Geometry check sheet. Reference: the model listing, model coordinates, mm. A direction names the side the tool comes from. Give positions to 0.01 mm unless a question says otherwise; leave off trailing zeros. Loops run counter-clockwise (first coordinate to the right, second up) from the corner with the lowest first, then second, coordinate; pieces in that order, holes last. Notation, with made-up numbers: (37.25, -17) -> (87.25, -17) arc R20 cw to (87.25, 15) -> close; hole circle Ø3 at (-28, 65). An arc over 180 degrees is marked (long way). One line per question, with ' | ' between items.
from build123d import *

# Parameters (mm, degrees)
ESQUISSE1_R                      = 2
ESQUISSE1_R_2                    = 1.8
ESQUISSE1_W                      = 7
ESQUISSE1_H                      = 9.3
ESQUISSE1_W_2                    = 9.3
ESQUISSE1_H_2                    = 7
BOSS_EXTRU_1_DEPTH               = 3
R_P_TITION_START                 = -3
R_P_TITION_CIRCULAIRE1_OUTLINE_R = 2
R_P_TITION_CIRCULAIRE1_DEPTH     = 6
CHANFREIN1_SIZE                  = 3
IDLER_REACH                      = 155.922
ESQUISSE2_R                      = 2.5
ESQUISSE2_W                      = 8
ESQUISSE2_H                      = 16
SCREEN_REACH                     = 155.922
ESQUISSE3_R                      = 2


# Read off the part's stored shape, not the designer's step: Répétition circulaire1
with BuildPart() as part:
    # Esquisse1 → Boss.-Extru.1 (new, symmetric)
    with BuildSketch(Plane.XY):
        with BuildLine():
            Line((-150, -26), (0, -26))
            Line((0, -26), (0, 26))
            Line((0, 26), (-4, 26))
            Line((-4, 26), (-4, 34))
            Line((-4, 34), (-81, 34))
            Line((-81, 34), (-81, 30))
            ThreePointArc((-81, 30), (-85, 26), (-89, 30))
            Line((-89, 30), (-89, 34))
            Line((-89, 34), (-98, 34))
            Line((-98, 34), (-98, 26))
            Line((-98, 26), (-118, 26))
            Line((-118, 26), (-118, 34))
            Line((-118, 34), (-150, 34))
            Line((-150, 34), (-150, -26))
        make_face()
        with Locations((-93, 28)):
            Circle(ESQUISSE1_R, mode=Mode.SUBTRACT)
        with Locations((-144, 4)):
            Circle(ESQUISSE1_R_2, mode=Mode.SUBTRACT)
        with Locations((-50, -20)):
            Circle(ESQUISSE1_R_2, mode=Mode.SUBTRACT)
        with Locations((-144, 15.65)):
            Rectangle(ESQUISSE1_W, ESQUISSE1_H, mode=Mode.SUBTRACT)
        with Locations((-144, -7.65)):
            Rectangle(ESQUISSE1_W, ESQUISSE1_H, mode=Mode.SUBTRACT)
        with Locations((-38.35, -20)):
            Rectangle(ESQUISSE1_W_2, ESQUISSE1_H_2, mode=Mode.SUBTRACT)
        with Locations((-61.65, -20)):
            Rectangle(ESQUISSE1_W_2, ESQUISSE1_H_2, mode=Mode.SUBTRACT)
    extrude(amount=BOSS_EXTRU_1_DEPTH, both=True)

    # Répétition circulaire1 outline → Répétition circulaire1 (cut)
    with BuildSketch(Plane.XY.offset(R_P_TITION_START)):
        with Locations((-77.07179677, 27.732050808)):
            Circle(R_P_TITION_CIRCULAIRE1_OUTLINE_R)
        with Locations((-85.138700708, 21.754955299)):
            Circle(R_P_TITION_CIRCULAIRE1_OUTLINE_R)
    extrude(amount=R_P_TITION_CIRCULAIRE1_DEPTH, mode=Mode.SUBTRACT)

    # Chanfrein1
    chanfrein1_edges = [part.edges().sort_by_distance(p)[0] for p in [
        (-118, 26, 0),
        (-98, 26, 0),
        (-4, 26, 0),
    ]]
    chamfer(chanfrein1_edges, length=CHANFREIN1_SIZE)

    # Symétrie2: part across plane


with BuildPart() as part_1:
    add(part.part)
    add(part.part.mirror(Plane(origin=(0, 26, 3), x_dir=(0, 0, 1), z_dir=(-1, 0, 0))))

    # Esquisse2 → idler (cut, up to next)
    with BuildSketch(Plane.XY.offset(3), mode=Mode.PRIVATE) as idler_sk1:
        with Locations((0, -10)):
            Circle(ESQUISSE2_R)
    idler_tool1 = extrude(idler_sk1.sketch, amount=-IDLER_REACH, mode=Mode.PRIVATE) & part_1.part
    # Esquisse2 → idler (cut, up to next)
    with BuildSketch(Plane.XY.offset(3), mode=Mode.PRIVATE) as idler_sk2:
        with Locations((-7, 6)):
            Rectangle(ESQUISSE2_W, ESQUISSE2_H)
    idler_tool2 = extrude(idler_sk2.sketch, amount=-IDLER_REACH, mode=Mode.PRIVATE) & part_1.part
    # Esquisse2 → idler (cut, up to next)
    with BuildSketch(Plane.XY.offset(3), mode=Mode.PRIVATE) as idler_sk3:
        with Locations((7, 6)):
            Rectangle(ESQUISSE2_W, ESQUISSE2_H)
    idler_tool3 = extrude(idler_sk3.sketch, amount=-IDLER_REACH, mode=Mode.PRIVATE) & part_1.part
    add(idler_tool1.solids().sort_by_distance((0, -10, 3))[0], mode=Mode.SUBTRACT)
    add(idler_tool2.solids().sort_by_distance((-7, 6, 3))[0], mode=Mode.SUBTRACT)
    add(idler_tool3.solids().sort_by_distance((7, 6, 3))[0], mode=Mode.SUBTRACT)

    # Esquisse3 → screen (cut, up to next)
    with BuildSketch(Plane.XY.offset(3), mode=Mode.PRIVATE) as screen_sk1:
        with Locations((-82.5, -11)):
            Circle(ESQUISSE3_R)
    screen_tool1 = extrude(screen_sk1.sketch, amount=-SCREEN_REACH, mode=Mode.PRIVATE) & part_1.part
    # Esquisse3 → screen (cut, up to next)
    with BuildSketch(Plane.XY.offset(3), mode=Mode.PRIVATE) as screen_sk2:
        with Locations((82.5, -11)):
            Circle(ESQUISSE3_R)
    screen_tool2 = extrude(screen_sk2.sketch, amount=-SCREEN_REACH, mode=Mode.PRIVATE) & part_1.part
    # Esquisse3 → screen (cut, up to next)
    with BuildSketch(Plane.XY.offset(3), mode=Mode.PRIVATE) as screen_sk3:
        Polygon((-59.999999802, -1), (-56.999999802, 2), (-42.999999802, 2), (-39.999999802, -1), (-39.999999802, -5), (-42.999999802, -8), (-56.999999802, -8), (-59.999999802, -5), align=None)
    screen_tool3 = extrude(screen_sk3.sketch, amount=-SCREEN_REACH, mode=Mode.PRIVATE) & part_1.part
    add(screen_tool1.solids().sort_by_distance((-82.5, -11, 3))[0], mode=Mode.SUBTRACT)
    add(screen_tool2.solids().sort_by_distance((82.5, -11, 3))[0], mode=Mode.SUBTRACT)
    add(screen_tool3.solids().sort_by_distance((-50, -3, 3))[0], mode=Mode.SUBTRACT)


solid = part_1.part
Item 1: Depth check by flat-ended pin: pin 1 Ø1.8 at (x, z) = (-106.5, -0.5) entering from +Y. Enter the tip coordinate at first touch or a pass-through.
Result:
pin 1: y = 26
Item 2: Sectioned sample at B-B (z = -1). Give the number of separate pieces and of enclosed holes in the cut face, plus the area to 3 significant figures.
Result:
separate pieces: 1 | enclosed holes: 24 | area: 16,400 mm2
Item 3: Release check for a two-part mould opening along X. For faces 3 (the face through (150, 4, 0)), 4 (the face through (-42, 34, 0)), 5 (the face through (98, 32, 0)) record: pulls with the +X half, pulls with the -X half, needs draft (parallel to the pull), parting line crosses it, or undercut.
Result:
face 3: pulls with the +X half | face 4: needs draft | face 5: undercut
Item 4: Sectioned sample at A-A (x = -108.5). Record the cut outline in (y, z).
Result:
outline: (-26, -3) -> (26, -3) -> (26, 3) -> (-26, 3) -> close
Item 5: Scan lines: probe 1 along X at (y, z) = (10, 0); probe 2 along Y at (x, z) = (-50, -0.9); probe 3 along X at (y, z) = (-17, -1). Record each from-to range of solid material in increasing order.
Result:
probe 1: -150 to -11, -3 to 3, 11 to 150 | probe 2: -26 to -21.8, -18.2 to -8, 2 to 34 | probe 3: -150 to -66.3, -57 to -43, -33.7 to 33.7, 43 to 57, 66.3 to 150
Item 6: Set-up check for faces 1 (the face through (4, 31, 0)), 2 (the face through (-147.5, 16, 0)): record each of +Z, -Z, +X, -X, +Y, -Y from which the full face is reachable in a straight line by a thin tool's end or side.
Result:
face 1: +Z, -Z, +Y | face 2: +Z, -Z
